Verification items for this drawing (mm, ordinates from the low corner). Round coordinates to 2 decimals unless told otherwise and drop trailing zeros. Order: outer loops, then holes, each group sorted by start corner. A loop starts at its lowest first (then second) coordinate and runs counter-clockwise, first axis right, second up.
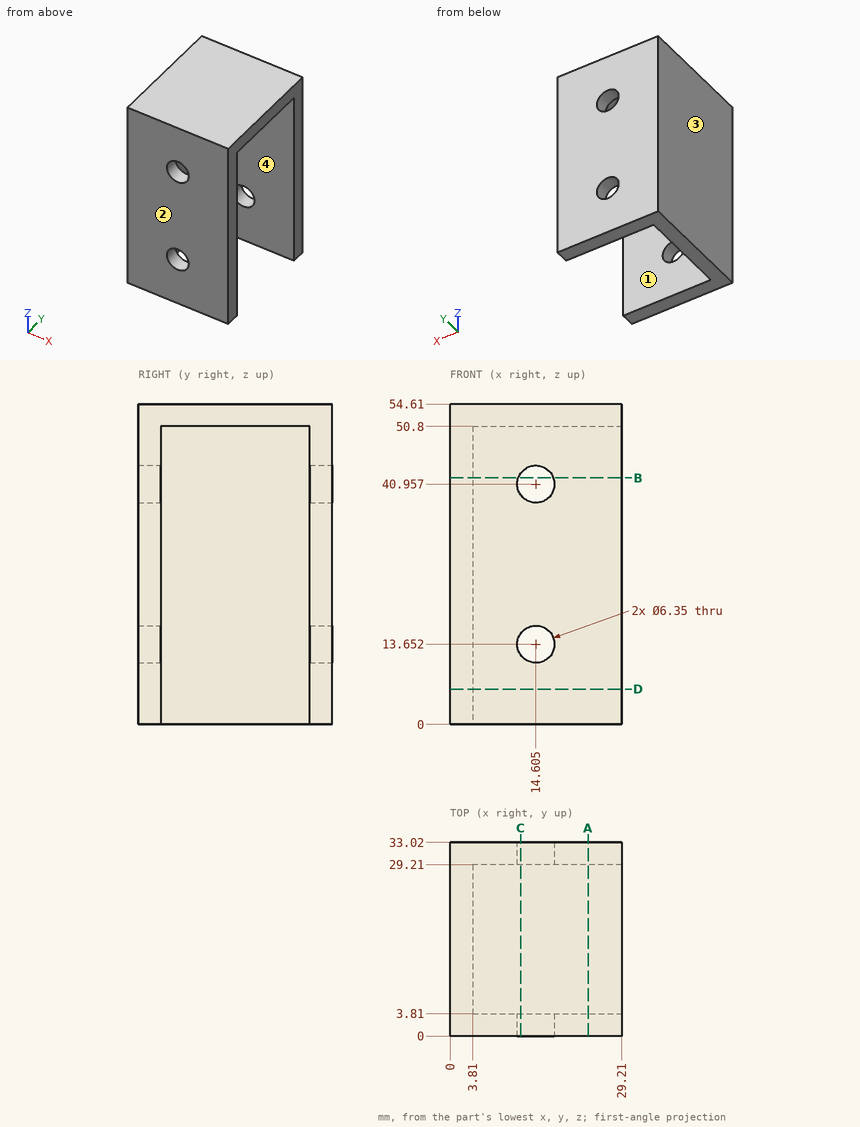
Item 1: Release check for a two-part mould opening along Y. For the marked faces 1, 2, 3 and 4 record: released by +Y, released by -Y, zero draft, split by the parting line, or undercut.
Answer:
face 1: undercut
face 2: released by -Y
face 3: zero draft
face 4: undercut
Item 2: Go/stop test with flat-tipped pins: P1, Ø2, axis at y = 6, z = 29, coming from the +X side; P2, Ø5, axis at x = 14.61, z = 40.96, coming from the -Y side; P3, Ø5, axis at x = 15.5, y = 19, coming from the -Z side. Record where each tip stops, or that it passes through.
Answer:
P1: stops at x = 3.81
P2: passes through
P3: stops at z = 50.8
Item 3: Sectioned sample at D-D (z = 6). Record the cut outline in (x, y).
Answer:
outline: (0, 0) - (29.21, 0) - (29.21, 3.81) - (3.81, 3.81) - (3.81, 29.21) - (29.21, 29.21) - (29.21, 33.02) - (0, 33.02) - close
Item 4: Scan lines: line 1 along Y through (x, z) = (16, 47); line 2 along Z through (x, y) = (16.25, 3) (1 decimal); line 3 along Z through (x, y) = (17, 25). Record each from-to range of solid material in increasing order.
Answer:
line 1: y = 0 to 3.81, 29.21 to 33.02
line 2: z = 0 to 10.9, 16.4 to 38.2, 43.7 to 54.6
line 3: z = 50.8 to 54.61
Item 5: Sectioned sample at A-A (x = 23.5). Record the cut outline in (y, z), and give its area (3 significant figures).
Answer:
outline: (0, 0) - (3.81, 0) - (3.81, 50.8) - (29.21, 50.8) - (29.21, 0) - (33.02, 0) - (33.02, 54.61) - (0, 54.61) - close
area: 513 mm2
Item 6: Sectioned sample at C-C (x = 12). Record the cut outline in (y, z).
Answer:
outline: (0, 0) - (3.81, 0) - (3.81, 11.84) - (0, 11.84) - close; (0, 15.47) - (3.81, 15.47) - (3.81, 39.14) - (0, 39.14) - close; (0, 42.77) - (3.81, 42.77) - (3.81, 50.8) - (29.21, 50.8) - (29.21, 42.77) - (33.02, 42.77) - (33.02, 54.61) - (0, 54.61) - close; (29.21, 0) - (33.02, 0) - (33.02, 11.84) - (29.21, 11.84) - close; (29.21, 15.47) - (33.02, 15.47) - (33.02, 39.14) - (29.21, 39.14) - close
Item 7: Sectioned sample at B-B (z = 42). Record the cut outline in (x, y).
Answer:
outline: (0, 0) - (11.61, 0) - (11.61, 3.81) - (3.81, 3.81) - (3.81, 29.21) - (11.61, 29.21) - (11.61, 33.02) - (0, 33.02) - close; (17.6, 0) - (29.21, 0) - (29.21, 3.81) - (17.6, 3.81) - close; (17.6, 29.21) - (29.21, 29.21) - (29.21, 33.02) - (17.6, 33.02) - close
